Geometry: final body of the model. Coordinates: model frame, mm. Face numbers are marked on the shaded views. A direction names the side the tool comes from. Give positions to 0.01 mm unless a question says otherwise; leave off trailing zeros. Order: outer loops, then holes, each group sorted by start corner. A loop starts at its lowest first (then second) coordinate and runs counter-clockwise, first axis right, second up. Notation, with made-up numbers: (85, -26) - (109, -26) arc R18 cw to (109, -8) - close; hole circle Ø9 at (-14, 85.25). An arc over 180 degrees is marked (long way). One line per item, written item: value.
```python
from build123d import *

# Parameters (mm, degrees)
F1_DEPTH = 16
F3_D     = 8
F5_D     = 8
F5_DEPTH = 8
F5_TIP   = 2.4034424761


with BuildPart() as f1:
    # F0 (on Front) → F1 (new body)
    with BuildSketch(Plane.XZ):
        Polygon((-8, -9.75), (8, -9.75), (8, 9.75), (4, 9.75), (4, 32.45), (0, 32.45), (-4, 32.45), (-4, 9.75), (-8, 9.75), align=None)
    extrude(amount=F1_DEPTH)

    # F3 (through all)
    with Locations(Plane.YZ.offset(4)):
        with Locations((-8, 21.95)):
            Hole(F3_D / 2)

    # F5
    with Locations(Plane(origin=(0, 0, -9.75), x_dir=(1, 0, 0), z_dir=(0, 0, -1))):
        with Locations((0, 8)):
            Hole(F5_D / 2, depth=F5_DEPTH)
            with Locations((0, 0, -(F5_DEPTH + F5_TIP / 2))):  # 118° drill point
                Cone(0, F5_D / 2, F5_TIP, mode=Mode.SUBTRACT)


solid = f1.part
```
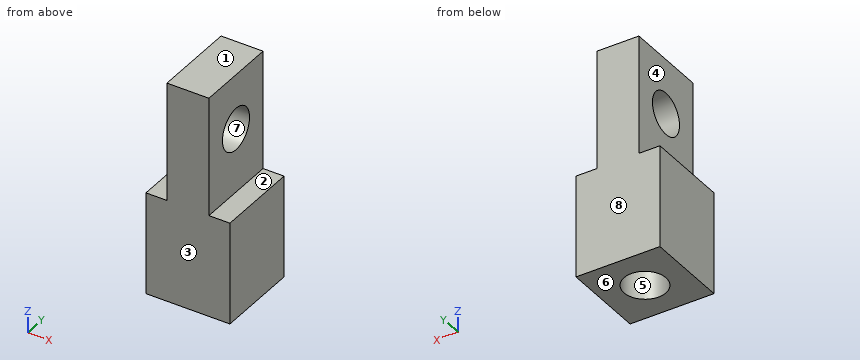
1) Section A-A, the plane z = 21.95. Return loops of the section in (x, y), then the cut area to 3 significant figures.
Answers below:
outline: (-4, -16) - (4, -16) - (4, -12) - (-4, -12) - close; (-4, -4) - (4, -4) - (4, 0) - (-4, 0) - close
area: 64.0 mm^2
2) Set-up query: the marked faces 1, 2, 3, 4 and 5. Return all of +Z, -Z, +X, -X, +Y, -Y with unobstructed straight access to the full face (end or side cutting, diameter ignored); none if empty.
Answers below:
face 1: +Z, +X, -X, +Y, -Y
face 2: +Z, +X, +Y, -Y
face 3: +Z, -Z, +X, -X, -Y
face 4: +Z, -X, +Y, -Y
face 5: -Z
3) Material intervals for line 1 along Y through (x, z) = (0, -7.5); line 2 along X through (y, z) = (-2.5, 17); line 3 along Z through (x, y) = (-7, -5.5), sorted ascending.
Answers below:
line 1: -16 to -12, -4 to 0
line 2: -4 to 4
line 3: -9.75 to 9.75
4) Section B-B, the plane x = -6.75. Return loops of the section in (y, z).
Answers below:
outline: (-16, -9.75) - (0, -9.75) - (0, 9.75) - (-16, 9.75) - close
5) Mould query, pull axis Y, two halves, no side actions, for the marked faces 6, 7 and 8. Classes: released by +Y, released by -Y, zero draft, split by the parting line, or undercut.
Answers below:
face 6: zero draft
face 7: undercut
face 8: released by +Y
6) First-contact query: pin 1 (3 mm diameter, centred on x = -4.5, z = 12.5, fed in from +Y); pin 2 (1.2 mm diameter, centred on x = 5.5, y = -6.5, fed in from +Z); pin 3 (9 mm diameter, centred on y = -8, z = 21.95, fed in from -X); pin 4 (7 mm diameter, centred on x = 0, y = -8, fed in from -Z). Flat tips, straight axial feed; report the tip coordinate or a pass-through.
Answers below:
pin 1: y = 0
pin 2: z = 9.75
pin 3: x = -4
pin 4: z = -1.45
